Study the drawing (mm; zero at the part's minimum x, y, z) and answer. A direction names the side the tool comes from. Coordinates: 2 decimals unless noted, no trailing zeros. Order: outer loops, then holes, each group sorted by start corner. A loop starts at its lowest first (then second) coordinate and runs counter-clockwise, first axis right, second up.
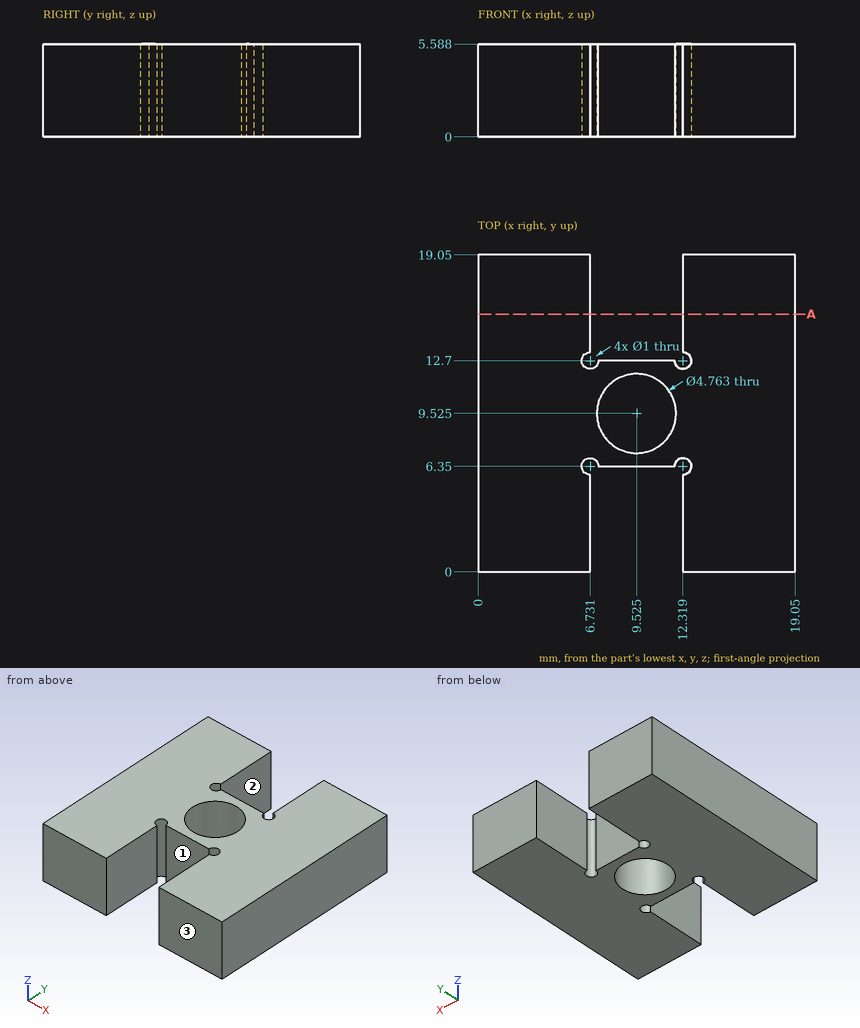
1) Straight lines are drawn through the part: line 1 (X direction, y = 16, z = 3.05); line 2 (X direction, y = 13, z = 3.05); line 3 (Y direction, x = 12, z = 1.3) (1 decimal). For each, find the intervals that lie inside material, in ascending order.
A:
line 1: x = 0 to 6.73, 12.32 to 19.05
line 2: x = 0 to 6.33, 12.72 to 19.05
line 3: y = 6.7 to 12.3
2) Flat-ended cylindrical pins translate along their axes: pin 1 Ø2.5 at (x, z) = (9, 1.5) entering from +Y; pin 2 Ø3 at (x, z) = (9.5, 4.5) entering from -Y. Find the tip coordinate at first contact, or state that the pin passes through.
A:
pin 1: stops at y = 12.7
pin 2: stops at y = 6.35
3) Which of the six approach directions +Z, -Z, +X, -X, +Y, -Y give full straight-line access (tool end or side, diameter ignored) to the marked faces 1, 2 and 3?
A:
face 1: +Z, -Z, -Y
face 2: +Z, -Z, +Y
face 3: +Z, -Z, +X, -X, -Y
4) A cutting plane is placed at A-A, the plane y = 15.5. Determine the outline of the cut face in (x, z).
A:
outline: (0, 0) - (6.73, 0) - (6.73, 5.59) - (0, 5.59) - close; (12.32, 0) - (19.05, 0) - (19.05, 5.59) - (12.32, 5.59) - close
